Input: part model. Units: mm. Frame: model coordinates. Coordinates: 2 decimals unless noted, no trailing zeros. Loops run counter-clockwise (first coordinate to the right, second up) from the corner with the lowest first, then second, coordinate; pieces in that order, holes last.
Item 1: Section D-D on y = 0.9. Give the number of separate pieces and of enclosed holes in the cut face, and give its area (3 significant figures).
Item 2: Section B-B on x = 41.5. Return loops of the section in (y, z).
Item 3: Section A-A on x = 33. Return loops of the section in (y, z), and give its area (3 significant figures).
Item 4: Section C-C on z = -3. Return loops of the section in (x, y), and give its area (3 significant figures).
Item 5: Ray query, line 1 along Z through (x, y) = (22.5, 1.2); line 2 along X through (y, z) = (1.35, -25); line 3 along Z through (x, y) = (12, 2.55). Return the intervals inside material, ascending.
```python
from build123d import *

# Parameters (mm, degrees)
SKETCH_1_W          = 45
SKETCH_1_H          = 28
EXTRUDE_1_DEPTH     = 3
SKETCH_2_R          = 1.25
SKETCH_2_W          = 7
SKETCH_2_H          = 3
CUT_EXTRUDE_1_DEPTH = 4
SKETCH_3_W          = 3
SKETCH_3_H          = 5
CUT_EXTRUDE_2_DEPTH = 4


with BuildPart() as part:
    # 스케치1 → 보스-돌출1 (new body)
    with BuildSketch(Plane(origin=(0, 0, 0), x_dir=(1, 0, 0), z_dir=(0, 1, 0))):
        with Locations((22.5, 14)):
            Rectangle(SKETCH_1_W, SKETCH_1_H)
    extrude(amount=EXTRUDE_1_DEPTH)

    # 스케치2 → 컷-돌출1 (cut, through all)
    with BuildSketch(Plane(origin=(0, 3, 0), x_dir=(1, 0, 0), z_dir=(0, 1, 0))):
        with Locations((22.5, 3)):
            Circle(SKETCH_2_R)
        with Locations((22.5, 25)):
            Circle(SKETCH_2_R)
        with Locations((3.5, 3)):
            Circle(SKETCH_2_R)
        with Locations((41.5, 3)):
            Circle(SKETCH_2_R)
        with Locations((41.5, 25)):
            Circle(SKETCH_2_R)
        with Locations((3.5, 25)):
            Circle(SKETCH_2_R)
        with Locations((32, 3)):
            Rectangle(SKETCH_2_W, SKETCH_2_H)
        with Locations((13, 3)):
            Rectangle(SKETCH_2_W, SKETCH_2_H)
        with Locations((32, 25)):
            Rectangle(SKETCH_2_W, SKETCH_2_H)
        with Locations((13, 25)):
            Rectangle(SKETCH_2_W, SKETCH_2_H)
    extrude(amount=-CUT_EXTRUDE_1_DEPTH, mode=Mode.SUBTRACT)

    # 스케치3 → 컷-돌출2 (cut, through all)
    with BuildSketch(Plane(origin=(0, 3, 0), x_dir=(1, 0, 0), z_dir=(0, 1, 0))):
        with Locations((11, 14)):
            Rectangle(SKETCH_3_W, SKETCH_3_H)
        with Locations((34, 14)):
            Rectangle(SKETCH_3_W, SKETCH_3_H)
    extrude(amount=-CUT_EXTRUDE_2_DEPTH, mode=Mode.SUBTRACT)


solid = part.part
```
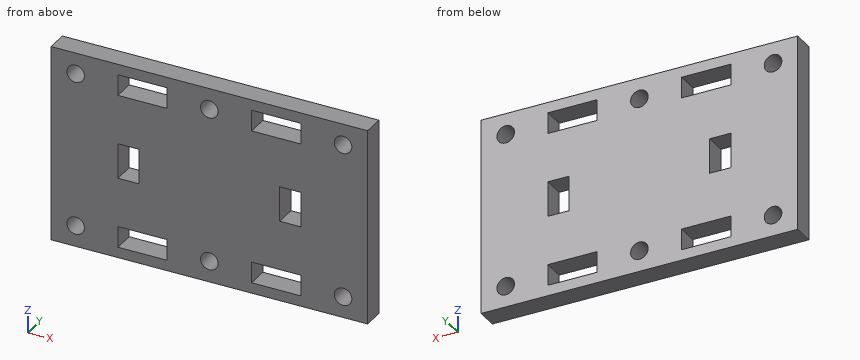
Results found:
1. separate pieces: 1
1. enclosed holes: 12
1. area: 1,120 mm2
2. outline: (0, -28) - (3, -28) - (3, -26.25) - (0, -26.25) - close; (0, -23.75) - (3, -23.75) - (3, -4.25) - (0, -4.25) - close; (0, -1.75) - (3, -1.75) - (3, 0) - (0, 0) - close
3. outline: (0, -28) - (3, -28) - (3, -26.5) - (0, -26.5) - close; (0, -23.5) - (3, -23.5) - (3, -16.5) - (0, -16.5) - close; (0, -11.5) - (3, -11.5) - (3, -4.5) - (0, -4.5) - close; (0, -1.5) - (3, -1.5) - (3, 0) - (0, 0) - close
3. area: 51.0 mm2
4. outline: (0, 0) - (2.25, 0) - (2.25, 3) - (0, 3) - close; (4.75, 0) - (9.5, 0) - (9.5, 3) - (4.75, 3) - close; (16.5, 0) - (21.25, 0) - (21.25, 3) - (16.5, 3) - close; (23.75, 0) - (28.5, 0) - (28.5, 3) - (23.75, 3) - close; (35.5, 0) - (40.25, 0) - (40.25, 3) - (35.5, 3) - close; (42.75, 0) - (45, 0) - (45, 3) - (42.75, 3) - close
4. area: 70.5 mm2
5. line 1: z = -28 to -26.25, -23.75 to -4.25, -1.75 to 0
5. line 2: x = 0 to 2.25, 4.75 to 9.5, 16.5 to 21.25, 23.75 to 28.5, 35.5 to 40.25, 42.75 to 45
5. line 3: z = -28 to -26.5, -23.5 to -16.5, -11.5 to -4.5, -1.5 to 0
